Check sheet for the drawn part. Datum: minimum x, y, z corner. Units: mm. A direction names the side the tool comes from. Give positions to 0.01 mm unless a question says otherwise; leave off trailing zeros. Order: outer loops, then holes, each group sorted by start corner. A loop starts at its lowest first (then second) coordinate and runs counter-clockwise, first axis right, second up. Notation, with made-up numbers: (47, -39) - (89, -39) arc R5 cw to (89, -30) - close; hole circle Ø3 at (-25.75, 84.5). An arc over 180 degrees is marked (long way). Answer as a JSON object with one key per item and string values. Group by question number.
(1) Section check A-A (y = 21). Record the boundary of the cut face in (x, z), then the cut area to 3 significant figures.
(2) Section check B-B (x = 128). Record the boundary of the cut face in (y, z).
(3) Depth check by flat-ended pin: pin 1 Ø4 at (x, z) = (111, 23) entering from -Y; pin 2 Ø1 at (y, z) = (50, 13) entering from +X; pin 3 Ø2 at (x, z) = (143, 25.5) entering from -Y. Enter the tip coordinate at first touch or a pass-through.
(4) Access from +Z, -Z, +X, -X, +Y, -Y to the whole of each face (thin tool, end or side, straight path). Record for the marked faces 1 and 2.
(5) Section check C-C (z = 18.25). Record the boundary of the cut face in (x, y).
(6) Thickness scan on line 1 (Y direction, x = 80, z = 27.5); line 2 (Y direction, x = 91, z = 14). Record the ranges inside material, lowest first.
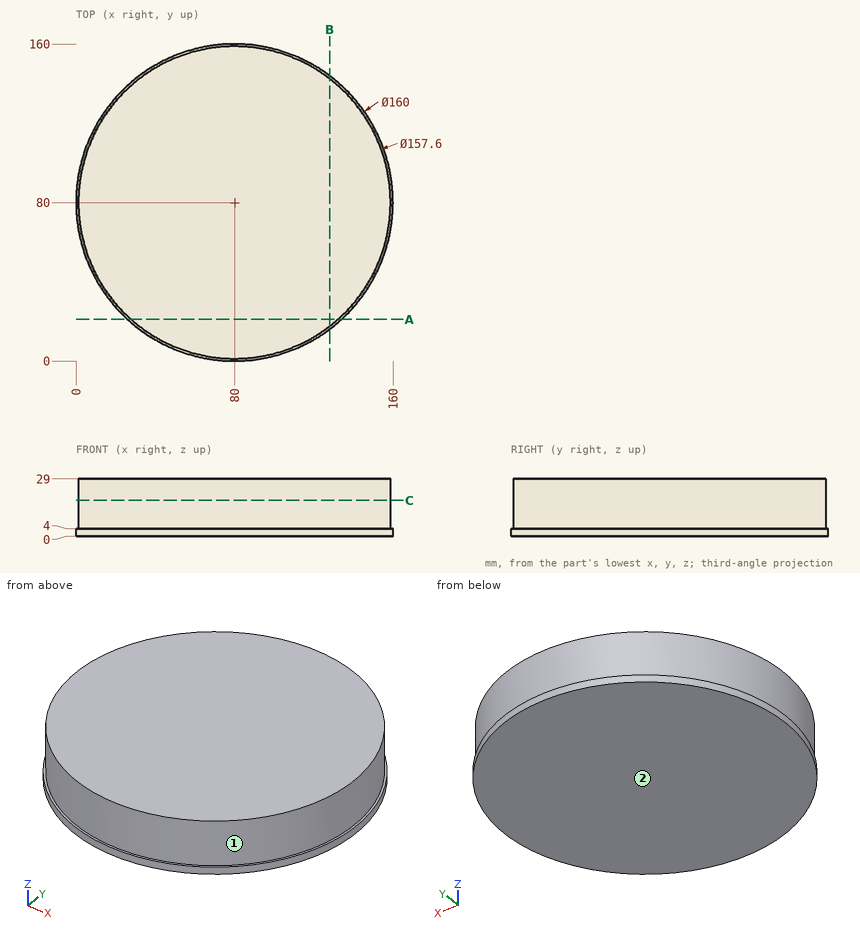
Solutions:
{
 "1": {"outline": "(25.97, 0) - (134.03, 0) - (134.03, 4) - (132.23, 4) - (132.23, 29) - (27.77, 29) - (27.77, 4) - (25.97, 4) - close", "area": "3,040 mm2"},
 "2": {"outline": "(16, 0) - (144, 0) - (144, 4) - (142.49, 4) - (142.49, 29) - (17.51, 29) - (17.51, 4) - (16, 4) - close"},
 "3": {"pin 1": "stops at y = 6.73", "pin 2": "stops at x = 153.07", "pin 3": "stops at y = 31.36"},
 "4": {"face 1": "+Z", "face 2": "-Z, +X, -X, +Y, -Y"},
 "5": {"outline": "circle Ø157.6 at (80, 80)"},
 "6": {"line 1": "y = 1.2 to 158.8", "line 2": "y = 1.97 to 158.03"}
}
